```python
from build123d import *

# Parameters (mm, degrees)
LINK_GEOMETRY_DEPTH                            = 30.572250038
SKETCH3_R                                      = 7.14375
JOINT_ROUNDS_DEPTH                             = 30.572250038
SKETCH5_R                                      = 2.38125
JOINT_HOLES_DEPTH                              = 323.793006671
SKETCH6_W                                      = 19.2375
SKETCH6_H                                      = 31.422524012
BULK_REMOVAL_DEPTH                             = 323.793006671
SKETCH7_W                                      = 19
SKETCH7_H                                      = 31.422524012
CONTACTPAD_OPENING_DEPTH                       = 217.555615914
SKETCH9_R                                      = 7.33425
CUT_EXTRUDE4_DEPTH                             = 3.286125
SKETCH12_W                                     = 53.268009521
SKETCH12_H                                     = 61.768223806
SURFACE_REDUCTION_DEPTH                        = 1.016
F_2_56_TAPPED_HOLE1_D                          = 1.778
F_2_56_TAPPED_HOLE1_CSINK_D                    = 5
F_2_56_TAPPED_HOLE1_CSINK_ANGLE                = 82
SKETCH19_R                                     = 7.33425
CUT_EXTRUDE8_DEPTH                             = 9.221875003
SKETCH20_W                                     = 21.352711571
SKETCH20_H                                     = 18.443750006
CUT_EXTRUDE9_DEPTH                             = 252.802485903
SKETCH21_W                                     = 24.193204712
SKETCH21_H                                     = 71.241054526
CUT_EXTRUDE10_DEPTH                            = 18.427750038
SKETCH22_R                                     = 0.535
CUT_EXTRUDE12_DEPTH                            = 18.427750038
SKETCH23_R                                     = 1.25
CUT_EXTRUDE13_DEPTH                            = 18.427750038
CUT_EXTRUDE14_DEPTH                            = 323.498364807
FILLET1_R                                      = 0.75
BOSS_EXTRUDE1_REACH                            = 320.899
SKETCH28_R                                     = 1.1303
PROX_SPRING_HOLE_DEPTH                         = 2.778125016
FILLET2_R                                      = 2.8
CSK_FOR_2_FLAT_HEAD_MACHINE_SCREW1_D           = 2.2606
CSK_FOR_2_FLAT_HEAD_MACHINE_SCREW1_DEPTH       = 2.777125016
CSK_FOR_2_FLAT_HEAD_MACHINE_SCREW1_CSINK_D     = 5.0999898
CSK_FOR_2_FLAT_HEAD_MACHINE_SCREW1_CSINK_ANGLE = 82
CSK_FOR_2_FLAT_HEAD_MACHINE_SCREW1_TIP         = 0.679152758
SKETCH32_R                                     = 1.025
DISTAL_SHEATH_HOLE_DEPTH                       = 19.05
DISTAL_SHEATH_SLOT_DEPTH                       = 19.05
FILLET3_R                                      = 3.175


with BuildPart() as part:
    # Sketch2 → link_geometry (new body)
    with BuildSketch(Plane.XY):
        Polygon((240.143856424, 163.499556409), (228.143856424, 151.378124535), (216.143856424, 156.973816433), (216.143856424, 193.282422523), (228.143856424, 206.378124535), (240.143856424, 204.262200767), align=None)
    extrude(amount=LINK_GEOMETRY_DEPTH)

    # Sketch3 → joint_rounds (add)
    with BuildSketch(Plane.XY.offset(30.572250038)):
        with Locations((228.143856424, 151.378124535)):
            Circle(SKETCH3_R)
        with Locations((228.143856424, 206.378124535)):
            Circle(SKETCH3_R)
    extrude(amount=-JOINT_ROUNDS_DEPTH)

    # Sketch5 → joint_holes (cut, through all)
    with BuildSketch(Plane.XY.offset(30.572250038)):
        with Locations((228.143856424, 206.378124535)):
            Circle(SKETCH5_R)
        with Locations((228.143856424, 151.378124535)):
            Circle(SKETCH5_R)
    extrude(amount=-JOINT_HOLES_DEPTH, mode=Mode.SUBTRACT)

    # Sketch6 → bulk_removal (cut, through all)
    with BuildSketch(Plane.XY.offset(30.572250038)):
        with Locations((230.525106424, 175.719125556)):
            Rectangle(SKETCH6_W, SKETCH6_H)
    extrude(amount=-BULK_REMOVAL_DEPTH, mode=Mode.SUBTRACT)

    # Sketch7 → contactpad_opening (cut, through all)
    with BuildSketch(Plane(origin=(220.906356424, 0, 0), x_dir=(0, 0, -1), z_dir=(1, 0, 0))):
        with Locations((-15.286125019, 175.719125556)):
            Rectangle(SKETCH7_W, SKETCH7_H)
    extrude(amount=-CONTACTPAD_OPENING_DEPTH, mode=Mode.SUBTRACT)

    # Sketch9 → Cut-Extrude4 (cut)
    with BuildSketch(Plane.XY.offset(30.572250038)):
        with Locations((228.143856424, 151.378124535)):
            Circle(SKETCH9_R)
        with Locations((228.143856424, 206.378124535)):
            Circle(SKETCH9_R)
    cut_extrude4 = extrude(amount=-CUT_EXTRUDE4_DEPTH, mode=Mode.SUBTRACT)

    # Sketch12 → surface_reduction (cut)
    with BuildSketch(Plane.ZY.offset(-216.143856424)):
        with Locations((15.227490437, 176.668068821)):
            Rectangle(SKETCH12_W, SKETCH12_H)
    extrude(amount=-SURFACE_REDUCTION_DEPTH, mode=Mode.SUBTRACT)

    # #2-56 Tapped Hole1 (through all)
    with Locations(Plane.ZY.offset(-217.159856424)):
        with Locations((2.893062509, 185.719125556), (2.893062509, 165.719125556), (27.679187528, 165.719125556), (27.679187528, 185.719125556)):
            CounterSinkHole(F_2_56_TAPPED_HOLE1_D / 2, F_2_56_TAPPED_HOLE1_CSINK_D / 2, counter_sink_angle=F_2_56_TAPPED_HOLE1_CSINK_ANGLE)

    # Sketch19 → Cut-Extrude8 (cut, symmetric)
    with BuildSketch(Plane.XY.offset(15.286125019)):
        with Locations((228.143856424, 206.378124535)):
            Circle(SKETCH19_R)
        with Locations((228.143856424, 151.378124535)):
            Circle(SKETCH19_R)
    extrude(amount=CUT_EXTRUDE8_DEPTH, both=True, mode=Mode.SUBTRACT)

    # Sketch20 → Cut-Extrude9 (cut, through all)
    with BuildSketch(Plane(origin=(0, 144.234374535, 0), x_dir=(-1, 0, 0), z_dir=(0, -1, 0))):
        with Locations((-231.58271221, -15.286125019)):
            Rectangle(SKETCH20_W, SKETCH20_H)
    extrude(amount=-CUT_EXTRUDE9_DEPTH, mode=Mode.SUBTRACT)

    # Sketch21 → Cut-Extrude10 (cut)
    with BuildSketch(Plane.XY.offset(27.286125038)):
        with Locations((233.00295878, 180.513642368)):
            Rectangle(SKETCH21_W, SKETCH21_H)
    cut_extrude10 = extrude(amount=CUT_EXTRUDE10_DEPTH, mode=Mode.SUBTRACT)

    # Mirror1: Cut-Extrude10 across plane
    add(cut_extrude10.mirror(Plane.XY.offset(15.286125019)), mode=Mode.SUBTRACT)

    # Mirror2: Cut-Extrude4 across plane
    add(cut_extrude4.mirror(Plane.XY.offset(15.286125019)), mode=Mode.SUBTRACT)

    # Sketch22 → Cut-Extrude12 (cut)
    with BuildSketch(Plane(origin=(98.729091699, 211.725220405, 0), x_dir=(0.906307787036652, -0.42261826174069506, 0), z_dir=(-0.42261826174069506, -0.906307787036652, 0))):
        with Locations((131.760393785, 15.286125019)):
            Circle(SKETCH22_R)
    extrude(amount=-CUT_EXTRUDE12_DEPTH, mode=Mode.SUBTRACT)

    # Sketch23 → Cut-Extrude13 (cut)
    with BuildSketch(Plane(origin=(99.39999819, 213.163984017, 0), x_dir=(0.906307787036652, -0.42261826174069506, 0), z_dir=(0.42261826174069506, 0.906307787036652, 0))):
        with Locations(Location((131.760393785, -15.286125019, 0), (0, 0, 48.607805398))):
            Circle(SKETCH23_R)
    extrude(amount=CUT_EXTRUDE13_DEPTH, mode=Mode.SUBTRACT)

    # Sketch25 → Cut-Extrude14 (cut, through all)
    with BuildSketch(Plane(origin=(0, 0, 3.286125), x_dir=(-1, 0, 0), z_dir=(0, 0, -1))):
        with BuildLine():
            Line((-220.906356424, 160.00786355), (-229.4639099, 158.398852623))
            ThreePointArc((-229.4639099, 158.398852623), (-231.462370725, 157.704310345), (-233.169757129, 156.454883952))
            Line((-233.169757129, 156.454883952), (-246.03003643, 156.454883952))
            Line((-246.03003643, 156.454883952), (-246.03003643, 205.137625366))
            Line((-246.03003643, 205.137625366), (-235.17907681, 205.137625366))
            ThreePointArc((-235.17907681, 205.137625366), (-234.289208718, 202.735624123), (-232.609215668, 200.801949243))
            Line((-232.609215668, 200.801949243), (-220.906356424, 191.430387562))
            Line((-220.906356424, 191.430387562), (-220.906356424, 160.00786355))
        make_face()
    extrude(amount=-CUT_EXTRUDE14_DEPTH, mode=Mode.SUBTRACT)

    # Fillet1
    fillet1_edges = [part.edges().sort_by_distance(p)[0] for p in [
        (220.906356424, 157.380444881, 6.064250016),
        (220.906356424, 194.955083411, 6.064250016),
        (220.906356424, 157.380444881, 24.508000022),
        (220.906356424, 194.955083411, 24.508000022),
        (220.906356424, 194.955083411, 27.286125038),
        (220.906356424, 157.380444881, 27.286125038),
        (220.906356424, 157.380444881, 3.286125),
        (220.906356424, 194.955083411, 3.286125),
    ]]
    fillet(fillet1_edges, radius=FILLET1_R)

    # Boss-Extrude1: up to this face of the body (flat: up to its plane)
    boss_extrude1_end = Plane(part.part.faces().sort_by_distance((221.752390309, 154.592187289, 6.064250016))[0])
    # Sketch26 → Boss-Extrude1 (add, up to the picked face)
    with BuildSketch(Plane(origin=(0, 0, 3.286125), x_dir=(-1, 0, 0), z_dir=(0, 0, -1)), mode=Mode.PRIVATE) as boss_extrude1_sk1:
        with BuildLine():
            Line((-220.906356424, 160.00786355), (-235.287606424, 160.00786355))
            Line((-235.287606424, 160.00786355), (-237.374220284, 160.00786355))
            Line((-237.374220284, 160.00786355), (-235.118271025, 149.831934043))
            ThreePointArc((-235.118271025, 149.831934043), (-234.106035024, 155.313298027), (-229.4639099, 158.398852623))
            Line((-229.4639099, 158.398852623), (-220.906356424, 160.00786355))
        make_face()
    boss_extrude1_tool1 = split(extrude(boss_extrude1_sk1.sketch, amount=-BOSS_EXTRUDE1_REACH, mode=Mode.PRIVATE), bisect_by=boss_extrude1_end, keep=Keep.BOTH, mode=Mode.PRIVATE)
    # Sketch26 → Boss-Extrude1 (add, up to the picked face)
    with BuildSketch(Plane(origin=(0, 0, 3.286125), x_dir=(-1, 0, 0), z_dir=(0, 0, -1)), mode=Mode.PRIVATE) as boss_extrude1_sk2:
        with BuildLine():
            Line((-220.906356424, 191.430387562), (-232.609215668, 200.801949243))
            ThreePointArc((-232.609215668, 200.801949243), (-234.583247525, 203.285002115), (-235.287606422, 206.377934686))
            Line((-235.287606422, 206.377934686), (-235.287209171, 191.430005382))
            Line((-235.287209171, 191.430005382), (-220.906356424, 191.430387562))
        make_face()
    boss_extrude1_tool2 = split(extrude(boss_extrude1_sk2.sketch, amount=-BOSS_EXTRUDE1_REACH, mode=Mode.PRIVATE), bisect_by=boss_extrude1_end, keep=Keep.BOTH, mode=Mode.PRIVATE)
    add(boss_extrude1_tool1.solids().sort_by(Axis((232.662189, 157.945837, 3.286125), (0, 0, 1)))[0])
    add(boss_extrude1_tool2.solids().sort_by(Axis((230.577028, 195.425201, 3.286125), (0, 0, 1)))[0])

    # Sketch28 → prox_spring_hole (cut)
    with BuildSketch(Plane(origin=(0, 0, 3.286125), x_dir=(-1, 0, 0), z_dir=(0, 0, -1))):
        with Locations((-233.769956424, 157.128124535)):
            Circle(SKETCH28_R)
        with Locations((-232.220400769, 194.605086885)):
            Circle(SKETCH28_R)
    extrude(amount=-PROX_SPRING_HOLE_DEPTH, mode=Mode.SUBTRACT)

    # Fillet2
    fillet2_edges = [part.edges().sort_by_distance(p)[0] for p in [
        (237.374220284, 160.00786355, 4.675187508),
    ]]
    fillet(fillet2_edges, radius=FILLET2_R)

    # CSK for #2 Flat Head Machine Screw1
    with Locations(Plane(origin=(0, 0, 3.286125), x_dir=(-1, 0, 0), z_dir=(0, 0, -1))):
        with Locations((-233.769956424, 157.128124535), (-232.220400769, 194.605086885)):
            CounterSinkHole(CSK_FOR_2_FLAT_HEAD_MACHINE_SCREW1_D / 2, CSK_FOR_2_FLAT_HEAD_MACHINE_SCREW1_CSINK_D / 2, depth=CSK_FOR_2_FLAT_HEAD_MACHINE_SCREW1_DEPTH, counter_sink_angle=CSK_FOR_2_FLAT_HEAD_MACHINE_SCREW1_CSINK_ANGLE)
            with Locations((0, 0, -(CSK_FOR_2_FLAT_HEAD_MACHINE_SCREW1_DEPTH + CSK_FOR_2_FLAT_HEAD_MACHINE_SCREW1_TIP / 2))):  # 118° drill point
                Cone(0, CSK_FOR_2_FLAT_HEAD_MACHINE_SCREW1_D / 2, CSK_FOR_2_FLAT_HEAD_MACHINE_SCREW1_TIP, mode=Mode.SUBTRACT)

    # Sketch32 → distal_sheath_hole (cut)
    with BuildSketch(Plane(origin=(22.676095468, -20.778813182, 0), x_dir=(0, 0, 1), z_dir=(-0.7372773368101212, 0.6755902076156635, 0))):
        with Locations(Location((15.286125019, 290.809071448, 0), (0, 0, 270))):
            Circle(SKETCH32_R)
    extrude(amount=-DISTAL_SHEATH_HOLE_DEPTH, mode=Mode.SUBTRACT)

    # Sketch33 → distal_sheath_slot (cut)
    with BuildSketch(Plane(origin=(22.676095468, -20.778813182, 0), x_dir=(0, 0, -1), z_dir=(0.7372773368101211, -0.6755902076156636, 0))):
        with BuildLine():
            Line((-15.936125019, 297.159071448), (-15.936125019, 284.459071448))
            ThreePointArc((-15.936125019, 284.459071448), (-15.286125019, 283.809071448), (-14.636125019, 284.459071448))
            Line((-14.636125019, 284.459071448), (-14.636125019, 297.159071448))
            ThreePointArc((-14.636125019, 297.159071448), (-15.286125019, 297.809071448), (-15.936125019, 297.159071448))
        make_face()
    extrude(amount=-DISTAL_SHEATH_SLOT_DEPTH, mode=Mode.SUBTRACT)

    # Fillet3
    fillet3_edges = [part.edges().sort_by_distance(p)[0] for p in [
        (235.287209171, 191.430005382, 4.675187508),
    ]]
    fillet(fillet3_edges, radius=FILLET3_R)


solid = part.part
```
Could you check a few things on this model? Use its own coordinates, in mm. A direction names the side the tool comes from. Round coordinates to 2 decimals unless told otherwise and drop trailing zeros. Loops run counter-clockwise (first coordinate to the right, second up) from the corner with the lowest first, then second, coordinate; pieces in that order, holes last. Notation, with made-up numbers: (-14.5, -17.5) -> (29.5, -17.5) arc R24 ccw to (29.5, -2.5) -> close; hole circle Ø1 at (-25.5, -27). An arc over 180 degrees is marked (long way). Put each result on its own line as item: value.
Q1. For pin 1 Ø4.5 at (x, y) = (227, 205) entering from +Z; pin 2 Ø1.7 at (y, z) = (187.5, 28.5) entering from +X; pin 3 Ø5 at (y, z) = (156, 25) entering from +X, each with a flat end and sliding along its axis, tell me the tip position at first contact or that it passes through.
Checks:
pin 1: z = 27.29
pin 2: x = 220.91
pin 3: x = 234.97
Q2. I want a section at A-A on z = 23. Write out the boundary of the cut face in (x, y).
Checks:
outline: (217.16, 156.5) -> (220.91, 154.75) -> (220.91, 160.01) -> (217.16, 160.01) -> close; (217.16, 191.43) -> (220.91, 191.43) -> (220.91, 198.48) -> (217.16, 194.39) -> close
Q3. Thinking about a two-plate mould opening in Y: for faces 1 (the flat face through (228, 154, 24.508)), 2 (the flat face through (235.88, 153.26, 4.66)), 3 (the cylindrical face through (234.332, 192.335, 4.695)), which applies, pulls with the +Y half, pulls with the -Y half, needs draft (parallel to the pull), parting line crosses it, or undercut?
Checks:
face 1: needs draft
face 2: pulls with the -Y half
face 3: undercut
Q4. I want a section at B-B on y = 170.5. Write out the boundary of the cut face in (x, z), and give its area (3 significant figures).
Checks:
outline: (217.16, 0) -> (220.91, 0) -> (220.91, 5.79) -> (217.16, 5.79) -> close; (217.16, 24.79) -> (220.91, 24.79) -> (220.91, 30.57) -> (217.16, 30.57) -> close
area: 43.4 mm2
Q5. I want a section at C-C on x = 222.5. Write out the boundary of the cut face in (y, z), and give its area (3 significant figures).
Checks:
outline: (147, 3.29) -> (160.01, 3.29) -> (160.01, 6.06) -> (147, 6.06) -> close; (147, 24.51) -> (159.71, 24.51) -> (159.71, 27.29) -> (147, 27.29) -> close; (191.43, 3.29) -> (200.22, 3.29) -> (200.22, 6.06) -> (191.43, 6.06) -> close; (192.71, 24.51) -> (200.22, 24.51) -> (200.22, 27.29) -> (192.71, 27.29) -> close; (202, 3.29) -> (210.76, 3.29) -> (210.76, 6.06) -> (202, 6.06) -> close; (202, 24.51) -> (210.76, 24.51) -> (210.76, 27.29) -> (202, 27.29) -> close
area: 165 mm2
Q6. Please list where these lines run through material, in increasing order: line 1 (Y direction, x = 226.5, z = 5.5); line 2 (Y direction, x = 222.25, z = 5); line 3 (Z direction, x = 220, y = 172). Write a range as from..to.
Checks:
line 1: 144.43..149.66, 153.1..160.01, 191.43..204.66, 208.1..213.33
line 2: 147.34..160.01, 191.43..199.95, 202.34..210.41
line 3: 0..5.79, 24.79..30.57
Q7. Which directions (+Z, -Z, +X, -X, +Y, -Y) give clear straight access to the entire face, cutting with the end or side of a thin tool? Please do faces 4 (the cylindrical face through (219.97, 184.85, 27.87)), 5 (the flat face through (219, 195, 14.636)), 6 (the flat face through (226.84, 196.18, 25.87)).
Checks:
face 4: +X, -X
face 5: -X, +Y
face 6: +Z, +X
